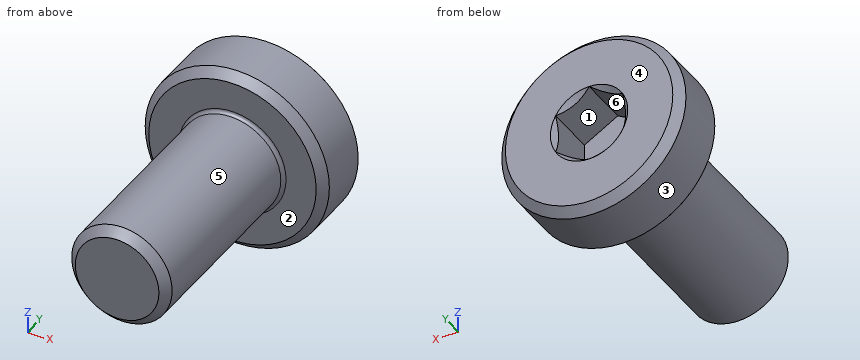
Autodesk Inventor part; units mm, degrees
ref_plane "YZ Plane" through (0, 0, 0) normal (1, 0, 0) x (0, 1, 0)
ref_plane "XZ Plane" through (0, 0, 0) normal (0, 1, 0) x (-1, 0, 0)
ref_plane "XY Plane" through (0, 0, 0) normal (0, 0, 1) x (1, 0, 0)
sketch "Sketch1" plane through (0, 0, 0) normal (0, 0, 1) x (1, 0, 0)
  line L0 (0, 4) -> (0, -4)
  line L1 (0, -4) -> (1.25, -4)
  line L2 (1.25, -4) -> (1.5, -3.75)
  line L3 (1.5, -3.75) -> (1.5, 1.9)
  line L4 (1.6, 2) -> (2.5, 2)
  line L5 (2.75, 2.25) -> (2.75, 3.75)
  line L6 (2.5, 4) -> (0, 4)
  arc A0 (1.6, 2) -> (1.5, 1.9) centre (1.6, 1.9) ccw
  line L7 (2.5, 4) -> (2.75, 3.75)
  line L8 (2.5, 2) -> (2.75, 2.25)
  point P0 (0, 0)
  point P1 (2.75, 2)
  point P2 (2.75, 4)
  point P3 (0, 0)
  dimension "d0" = 5.5
  dimension "d1" = 2
  dimension "d3" = 3
  dimension "d4" = 3.2
  dimension "d5" = 135
  dimension "d6" = 0.25
  dimension "d7" = 6
  dimension "d9" = 0.25
revolve "Revolution1" add sketch "Sketch1" angle 360 about axis through (0, 4, 0) along (0, -1, 0)
sketch "Sketch2" plane through (0, 4, 0) normal (0, 1, 0) x (1, 0, 0)
  line L0 (0, -1.1547) -> (-1, -0.5774)
  line L1 (-1, -0.5774) -> (-1, 0.5774)
  line L2 (-1, 0.5774) -> (0, 1.1547)
  line L3 (0, 1.1547) -> (1, 0.5774)
  line L4 (1, 0.5774) -> (1, -0.5774)
  line L5 (1, -0.5774) -> (0, -1.1547)
  point P0 (0, 0)
  point P1 (0, 0)
  dimension "d11" = 2
extrude "Extrusion1" cut sketch "Sketch2" against normal blind 1.5
thread "Thread1"
sketch "Sketch3" plane through (0, 0, 0) normal (1, 0, 0) x (0, 1, 0)
  line L0 (4, 1.1547) -> (3, 0.1547)
  line L1 (3, 0.1547) -> (4, 0.1547)
  line L2 (4, 0.1547) -> (4, 1.1547)
  line L3 (-0.8, 0) -> (4.8, 0)
  point P0 (0, 0)
  dimension "d18" = 1
revolve "Revolution2" cut sketch "Sketch3" angle 360 about axis through (0, -10, 0) along (0, 1, 0)
properties part number "Bolt_M3x0.35_6mm_SH" material "Stainless Steel"
Could you check a few things on this model? Use its own coordinates, in mm. Face numbers are marked on the shaded views. A direction names the side the tool comes from. Round coordinates to 2 decimals unless told otherwise and drop trailing zeros. Order: outer loops, then holes, each group sorted by start corner. A loop starts at its lowest first (then second) coordinate and runs counter-clockwise, first axis right, second up.
(1) Imagine slicing it at A-A (z = 0). Write out the boundary of the cut face in (x, y), plus the area to 3 significant figures.
Response values:
outline: (-2.75, 2.25) - (-2.5, 2) - (-1.6, 2) arc R0.1 cw to (-1.5, 1.9) - (-1.5, -3.75) - (-1.25, -4) - (1.25, -4) - (1.5, -3.75) - (1.5, 1.9) arc R0.1 cw to (1.6, 2) - (2.5, 2) - (2.75, 2.25) - (2.75, 3.75) - (2.5, 4) - (1.15, 4) - (1, 3.85) - (1, 2.5) - (-1, 2.5) - (-1, 3.85) - (-1.15, 4) - (-2.5, 4) - (-2.75, 3.75) - close
area: 25.8 mm2
(2) If we mould it in two halves opening along Z, with no side actions, what happens to the marked faces 4, 5 and 6? For each: released by +Z, released by -Z, zero draft, split by the parting line, or undercut.
Response values:
face 4: zero draft
face 5: split by the parting line
face 6: undercut
(3) I'm going to push flat-ended pins straight in: pin 1 (0.6 mm diameter, centred on x = -0.5, z = 0, fed in from +Y); pin 2 (1.5 mm diameter, centred on y = -0.5, z = -1.5, fed in from -X). Where does each tip first touch, or does it pass through?
Response values:
pin 1: stops at y = 2.5
pin 2: stops at x = -1.3
(4) Imagine slicing it at B-B (y = -0.25). Write out the boundary of the cut face in (x, z), plus the area to 3 significant figures.
Response values:
outline: circle Ø3 at (0, 0)
area: 7.07 mm2
(5) Which directions (+Z, -Z, +X, -X, +Y, -Y) give clear straight access to the entire face, cutting with the end or side of a thin tool? Please do the marked faces 1, 2 and 3.
Response values:
face 1: +Y
face 2: -Y
face 3: +Y, -Y
(6) Please list where these lines run through material, in increasing order: line 1 along Y through (x, z) = (1.35, -1.4); line 2 along Y through (x, z) = (0.2, -0.9); line 3 along Z through (x, y) = (0.5, -1.5).
Response values:
line 1: y = 2 to 4
line 2: y = -4 to 2.5
line 3: z = -1.41 to 1.41
